Here's how the part is built. I have some questions about the finished solid (model axes, mm). A direction names the side the tool comes from. Round coordinates to 2 decimals unless told otherwise and drop trailing zeros. Loops run counter-clockwise (first coordinate to the right, second up) from the corner with the lowest first, then second, coordinate; pieces in that order, holes last. Notation, with made-up numbers: M 39.25,-26 L 63.25,-26 A14 ccw 63.25,-8 Z; hole C 48.25,57 d10. An arc over 180 degrees is marked long. Answer as a JSON object with one key per item and string values.
from build123d import *

# Parameters (mm, degrees)
BOSS_EXTRUDE1_DEPTH = 3.175


with BuildPart() as part:
    # Sketch1 → Boss-Extrude1 (new body)
    with BuildSketch(Plane(origin=(0, 0, 0), x_dir=(1, 0, 0), z_dir=(0, 1, 0))):
        with BuildLine():
            Line((-36.784871939, 0), (-23.8125, 0))
            Line((-23.8125, 0), (-23.8125, 3.175))
            Line((-23.8125, 3.175), (-14.2875, 3.175))
            Line((-14.2875, 3.175), (-14.2875, 0))
            Line((-14.2875, 0), (-4.7625, 0))
            Line((-4.7625, 0), (-4.7625, 3.175))
            Line((-4.7625, 3.175), (4.7625, 3.175))
            Line((4.7625, 3.175), (4.7625, 0))
            Line((4.7625, 0), (14.2875, 0))
            Line((14.2875, 0), (14.2875, 3.175))
            Line((14.2875, 3.175), (23.8125, 3.175))
            Line((23.8125, 3.175), (23.8125, 0))
            Line((23.8125, 0), (36.784871939, 0))
            ThreePointArc((36.784871939, 0), (37.999891837, -0.241682484), (39.02993597, -0.92993597))
            Line((39.02993597, -0.92993597), (66.469065694, -28.369065694))
            ThreePointArc((66.469065694, -28.369065694), (66.920159512, -32.290840151), (63.203219493, -33.620560958))
            Line((63.203219493, -33.620560958), (1.5875, -12.7))
            Line((1.5875, -12.7), (1.5875, -6.35))
            Line((1.5875, -6.35), (-1.5875, -6.35))
            Line((-1.5875, -6.35), (-1.5875, -12.7))
            Line((-1.5875, -12.7), (-63.203219493, -33.620560958))
            ThreePointArc((-63.203219493, -33.620560958), (-66.920159512, -32.290840151), (-66.469065694, -28.369065694))
            Line((-66.469065694, -28.369065694), (-39.02993597, -0.92993597))
            ThreePointArc((-39.02993597, -0.92993597), (-37.999891837, -0.241682484), (-36.784871939, 0))
        make_face()
        with BuildLine():
            Line((-39.452913677, -18.850511262), (-9.014608915, -8.515706841))
            ThreePointArc((-9.014608915, -8.515706841), (-8.234573307, -7.9371291), (-7.9375, -7.012491225))
            Line((-7.9375, -7.012491225), (-7.9375, -6.35))
            Line((-7.9375, -6.35), (-34.154615818, -6.35))
            ThreePointArc((-34.154615818, -6.35), (-35.369635716, -6.591682484), (-36.399679849, -7.27993597))
            Line((-36.399679849, -7.27993597), (-42.718759878, -13.599015999))
            ThreePointArc((-42.718759878, -13.599015999), (-43.169853696, -17.520790456), (-39.452913677, -18.850511262))
        make_face(mode=Mode.SUBTRACT)
        with BuildLine():
            Line((39.452913677, -18.850511262), (9.014608915, -8.515706841))
            ThreePointArc((9.014608915, -8.515706841), (8.234573307, -7.9371291), (7.9375, -7.012491225))
            Line((7.9375, -7.012491225), (7.9375, -6.35))
            Line((7.9375, -6.35), (34.154615818, -6.35))
            ThreePointArc((34.154615818, -6.35), (35.369635716, -6.591682484), (36.399679849, -7.27993597))
            Line((36.399679849, -7.27993597), (42.718759878, -13.599015999))
            ThreePointArc((42.718759878, -13.599015999), (43.169853696, -17.520790456), (39.452913677, -18.850511262))
        make_face(mode=Mode.SUBTRACT)
    extrude(amount=BOSS_EXTRUDE1_DEPTH)


solid = part.part
Item 1: I want a section at D-D on y = 2.5. Count the separate pieces of the cut face and the enclosed holes in it, plus the area to 3 significant figures.
Solution:
{"separate pieces": "1", "enclosed holes": "2", "area": "1,900 mm2"}
Item 2: I want a section at C-C on z = 10. List the corners of the cut face in (x, y) for me (1 decimal).
Solution:
{"outline": "M -48.1,0 L -39.1,0 L -39.1,3.2 L -48.1,3.2 Z; M -13.4,0 L -1.6,0 L -1.6,3.2 L -13.4,3.2 Z; M 1.6,0 L 13.4,0 L 13.4,3.2 L 1.6,3.2 Z; M 39.1,0 L 48.1,0 L 48.1,3.2 L 39.1,3.2 Z"}
Item 3: For faces 1 (the face through (-30, 2, 0)), 2 (the face through (-31.964, 1.565, 23.014)), 3 (the face through (-4.762, 2, -2)), which set-ups out of +Z, -Z, +X, -X, +Y, -Y let a thin tool reach every point of the face, with its end or its side?
Solution:
{"face 1": "-Z, -X, +Y, -Y", "face 2": "+Z, +Y, -Y", "face 3": "-Z, +Y, -Y"}
Item 4: We'd pull the mould along X, two halves only. Please class faces 4 (the face through (-19, 2, -3.175)), 5 (the face through (32.827, 1.565, 23.307)), 6 (the face through (23.812, 2, -2)): +X half, -X half, draft (parallel to the pull), parting line (faces both ways), or undercut.
Solution:
{"face 4": "draft", "face 5": "undercut", "face 6": "+X half"}
Item 5: For P1, Ø1, axis at y = 1.5, z = -1.5, coming from the +X side; P2, Ø1.5, axis at x = -41.5, y = 2, coming from the -Z side; P3, Ø1, axis at y = 1.5, z = 10.5, coming from the +X side, each with a flat end and sliding along its axis, tell me the tip position at first contact or that it passes through.
Solution:
{"P1": "stops at x = 23.81", "P2": "stops at z = 2.65", "P3": "stops at x = 49.1"}
Item 6: If I drill on L1, parallel to X at y = 0.65, z = -0.5; L2, parallel to Z at x = 41, y = 1.3; L3, parallel to Z at x = 40, y = 1.75, over which ranges is the centre line in solid material (lowest first)? Write a range as from..to.
Solution:
{"L1": "x = -23.81..-14.29, -4.76..4.76, 14.29..23.81", "L2": "z = 2.9..11.88, 18.98..26.08", "L3": "z = 1.9..10.88, 18.98..25.74"}
Item 7: I want a section at B-B on x = 16.5. List the corners of the cut face in (y, z) for me (3 decimals), plus the area to 3 significant figures.
Solution:
{"outline": "M 0,-3.175 L 3.175,-3.175 L 3.175,6.35 L 0,6.35 Z; M 0,11.057 L 3.175,11.057 L 3.175,17.763 L 0,17.763 Z", "area": "51.5 mm2"}
Item 8: I want a section at A-A on z = 25. List the corners of the cut face in (x, y) for me (3 decimals), plus the area to 3 significant figures.
Solution:
{"outline": "M -63.1,0 L -37.814,0 L -37.814,3.175 L -63.1,3.175 Z; M 37.814,0 L 63.1,0 L 63.1,3.175 L 37.814,3.175 Z", "area": "161 mm2"}
